Geometry: see drawing. Coordinates: mm, zero at the bounding-box minimum. A direction names the side the tool comes from. Give positions to 0.01 mm unless a question says otherwise; leave off trailing zeros. Order: outer loops, then holes, each group sorted by start corner. A loop starts at its lowest first (then second) coordinate and runs counter-clockwise, first axis right, second up. Notation, with made-up numbers: M 47,-9.75 L 82,-9.75 A7 ccw 82,-2.75 Z; hole C -19.5,7.5 d3. An arc over 180 degrees is marked long. Write item = value, one per line. Start each with the question number.
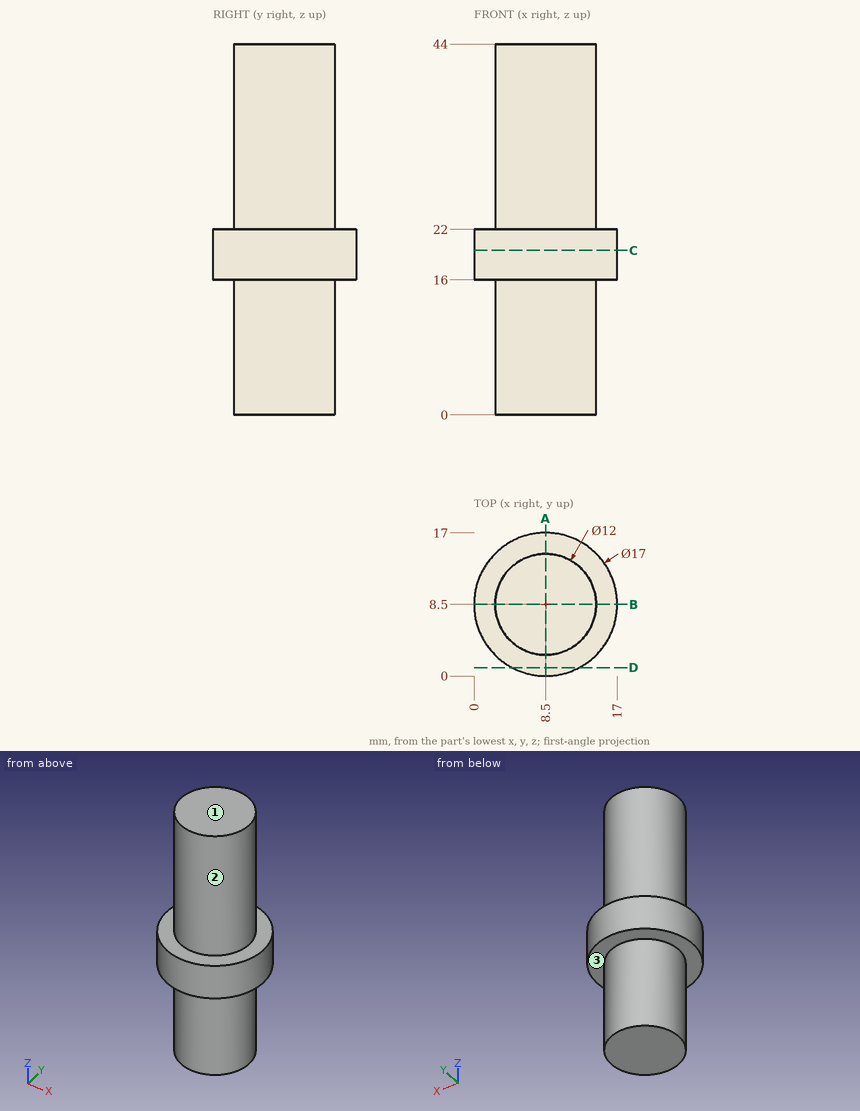
1) Cut plane D-D (y = 1). Return loops of the section in (x, z).
2) Access query for the marked faces 1, 2 and 3. Directions: +Z, -Z, +X, -X, +Y, -Y. A direction counts if a zero-diameter tool reaches every point of the face in a straight line with its end or side. Return the directions, or none.
3) Cut plane A-A (x = 8.5). Return loops of the section in (y, z).
4) Cut plane C-C (z = 19.5). Return loops of the section in (x, y), plus the area to 3 significant figures.
5) Ray query, L1, parallel to Z at x = 14.25, y = 3.75; L2, parallel to Y at x = 10.5, z = 12; L3, parallel to X at y = 9.25, z = 32. Return the intervals inside material, ascending.
6) Pin query (flat end, axial travel): pin 1 Ø2 at (x, z) = (9, 25.5) entering from -Y; pin 2 Ø1.5 at (x, z) = (10.5, 21.5) entering from -Y; pin 3 Ø1 at (x, y) = (5.5, 15) entering from -Z. Return the tip coordinate at first contact, or that it passes through.
Reply:
q1.outline = M 4.5,16 L 12.5,16 L 12.5,22 L 4.5,22 Z
q2.face_1 = +Z, +X, -X, +Y, -Y
q2.face_2 = +Z
q2.face_3 = -Z
q3.outline = M 0,16 L 2.5,16 L 2.5,0 L 14.5,0 L 14.5,16 L 17,16 L 17,22 L 14.5,22 L 14.5,44 L 2.5,44 L 2.5,22 L 0,22 Z
q4.outline = C 8.5,8.5 d17
q4.area = 227 mm²
q5.L1 = 16 to 22
q5.L2 = 2.84 to 14.16
q5.L3 = 2.55 to 14.45
q6.pin_1 = 2.5
q6.pin_2 = 0.09
q6.pin_3 = 16
